Autodesk Fusion 360 part; units mm, degrees
sketch "Sketch1" plane through (0, 0, 0) normal (0, 0, 1) x (1, 0, 0)
  line L0 (0, 25) -> (5, 25)
  line L1 (5, 25) -> (5, 5)
  line L2 (5, 0) -> (0, 0)
  line L3 (0, 0) -> (0, 25)
  line L4 (0, 0) -> (25, 0)
  line L5 (25, 0) -> (25, 5)
  line L6 (25, 5) -> (5, 5)
  line L7 (0, 5) -> (0, 0)
  dimension "d1" = 5
  dimension "d6" = 5
  dimension "d7" = 25
  dimension "d8" = 25
extrude "Extrude1" add sketch "Sketch1" along normal blind 100
sketch "Sketch2" plane through (0, 5, 0) normal (0, 1, 0) x (-1, 0, 0)
  line L0 (-25, 0) -> (-5, 0)
  line L1 (-5, 0) -> (-5, 100)
  line L2 (-5, 100) -> (-25, 100)
  line L3 (-25, 100) -> (-25, 0)
  circle A0 centre (-15, 70) radius 6.25
  circle A1 centre (-15, 50) radius 6.25
  circle A2 centre (-15, 30) radius 6.25
  line L4 (0, 0) -> (0, 100)
  dimension "d12" = 12.5
  dimension "d13" = 12.5
  dimension "d14" = 12.5
  dimension "d15" = 20
  dimension "d16" = 20
  dimension "d17" = 30
  dimension "d19" = 10
  dimension "d20" = 10
  dimension "d21" = 10
  dimension "d22" = 30
  dimension "d48" = 15
extrude "Extrude2" cut sketch "Sketch2" against normal blind 10 contours A0 | A1 | A2
sketch "Sketch3" plane through (5, 0, 0) normal (1, 0, 0) x (0, 1, 0)
  line L0 (5, 0) -> (25, 0)
  line L1 (25, 0) -> (25, 100)
  line L2 (25, 100) -> (5, 100)
  line L3 (5, 100) -> (5, 0)
  circle A0 centre (15, 10) radius 1.5
  circle A1 centre (15, 50) radius 1.5
  circle A2 centre (15, 90) radius 1.5
  dimension "d25" = 3
  dimension "d26" = 3
  dimension "d27" = 3
  dimension "d28" = 10
  dimension "d29" = 40
  dimension "d30" = 40
  dimension "d32" = 10
  dimension "d33" = 10
  dimension "d34" = 10
  dimension "d35" = 10
extrude "Extrude3" cut sketch "Sketch3" against normal blind 10 contours A0 | A1 | A2
fillet "Fillet1" radius 1 1 edges at (5, 5, 50)
fillet "Fillet2" radius 5 1 edges at (2.5, 25, 100)
fillet "Fillet3" radius 5 1 edges at (25, 2.5, 100)
fillet "Fillet4" radius 5 1 edges at (2.5, 25, 0)
fillet "Fillet5" radius 5 1 edges at (25, 2.5, 0)
Design review of the part built by this model. Coordinates are the model's own, in mm. A direction names the side the tool comes from. Coordinates: 2 decimals unless noted, no trailing zeros. Loops run counter-clockwise (first coordinate to the right, second up) from the corner with the lowest first, then second, coordinate; pieces in that order, holes last. Notation, with made-up numbers: (45.5, 77) - (54.5, 77) arc R13 ccw to (54.5, 86) - close; hole circle Ø8 at (55.25, 78). An arc over 180 degrees is marked (long way). Use CSV: the item, a comma, the result in double quotes. Start each with the question number.
1) Consider section B-B on z = 30. Write out the cut boundary in (x, y).
2) Consider section D-D on z = 82.5. Write out the cut boundary in (x, y), then the cut area to 3 significant figures.
3) Wall thickness on L1, parallel to Z at x = 15, y = 3.4; L2, parallel to Z at x = 2.45, y = 15; L3, parallel to Y at x = 2, z = 90: over which ranges is each line inside the solid? List them lowest first. Write a range as from..to.
4) Consider section C-C on y = 2. Write out the cut boundary in (x, z).
5) Consider section A-A on z = 50. Write out the cut boundary in (x, y).
6) The part is to be moulded in two halves that separate along X. For faces 3 (the flat face through (2, 25, 49)), 4 (the cylindrical face through (15.8, 2.5, 56.2)), 5 (the cylindrical face through (15.8, 2.5, 76.2)), 6 (the flat face through (25, 2, 49)), say which applies: +X half, -X half, draft (parallel to the pull), parting line (faces both ways), or undercut.
7) For pin 1 Ø5 at (y, z) = (15, 90) entering from +X; pin 2 Ø12 at (x, z) = (15, 20.5) entering from +Y, all flat-tipped, find the tip position at first contact; note any pin that passes through.
8) Tool access review of faces 1 (the cylindrical face through (3, 24, 98)), 2 (the flat face through (5, 18, 49)): name each direction out of +Z, -Z, +X, -X, +Y, -Y from which nothing blocks a thin tool from reaching the whole face with its end or side.
Geometry says:
1,outline,"(0, 0) - (8.75, 0) - (8.75, 5) - (6, 5) arc R1 cw to (5, 6) - (5, 25) - (0, 25) - close; (21.25, 0) - (25, 0) - (25, 5) - (21.25, 5) - close"
2,outline,"(0, 0) - (25, 0) - (25, 5) - (6, 5) arc R1 cw to (5, 6) - (5, 25) - (0, 25) - close"
2,area,"225 mm^2"
3,L1,"0..23.75, 36.25..43.75, 56.25..63.75, 76.25..100"
3,L2,"0..8.5, 11.5..48.5, 51.5..88.5, 91.5..100"
3,L3,"0..13.5, 16.5..25"
4,outline,"(0, 0) - (20, 0) arc R5 ccw to (25, 5) - (25, 95) arc R5 ccw to (20, 100) - (0, 100) - close; hole circle Ø12.5 at (15, 30); hole circle Ø12.5 at (15, 50); hole circle Ø12.5 at (15, 70)"
5,outline,"(0, 0) - (8.75, 0) - (8.75, 5) - (6, 5) arc R1 cw to (5, 6) - (5, 13.5) - (0, 13.5) - close; (0, 16.5) - (5, 16.5) - (5, 25) - (0, 25) - close; (21.25, 0) - (25, 0) - (25, 5) - (21.25, 5) - close"
6,face 3,"draft"
6,face 4,"undercut"
6,face 5,"undercut"
6,face 6,"+X half"
7,pin 1,"x = 5"
7,pin 2,"y = 5"
8,face 1,"+Z, +X, -X, +Y"
8,face 2,"+Z, -Z, +X, +Y"
